Here's how the part is built. I have some questions about the finished solid (model axes, mm). A direction names the side the tool comes from. Round coordinates to 2 decimals unless told otherwise and drop trailing zeros. Write each loop counter-clockwise with the first axis right and the second up, starting at its lowest first coordinate (ties: lowest second). Pieces come first, ordered by that corner, then holes. Notation, with made-up numbers: (-27, 36.5) - (15, 36.5) arc R13 cw to (15, 49.5) - close; hole circle Ø3 at (1, 21.5). An arc over 180 degrees is marked (long way). One line per question, with ' | ' between items. Start each with the question number.
(1) Imagine slicing it at C-C (y = 147). Write out the boundary of the cut face in (x, z), plus the area to 3 significant figures.
(2) For faces 1 (the flat face through (30, 142, 24)), 2 (the flat face through (29, 149, 42)), 3 (the flat face through (32, -5, 45)), 4 (the flat face through (32, 147, 45)), which set-ups out of +Z, -Z, +X, -X, +Y, -Y let a thin tool reach every point of the face, with its end or its side?
(3) Imagine slicing it at D-D (z = 32). Write out the boundary of the cut face in (x, y), plus the area to 3 significant figures.
(4) Imagine slicing it at B-B (x = 29). Give the number of separate pieces and of enclosed holes in the cut face, plus the area to 3 significant figures.
(5) Will these pins go through, and if not, where does the flat tip stop? pin 1 (10 mm diameter, centred on x = 37.5, z = 42, fed in from +Y); pin 2 (3.5 mm diameter, centred on x = 29, y = 147, fed in from +Z); pin 3 (6 mm diameter, centred on x = 14, z = 15.5, fed in from -Y); pin 4 (1 mm diameter, centred on y = 89, z = 21, fed in from -X).
(6) Thinking about a two-plate mould opening in Y: for faces 5 (the flat face through (26, 147, 44)), 6 (the flat face through (30, -2, 23)), 7 (the flat face through (60, 72, 24)), which applies, pulls with the +Y half, pulls with the -Y half, needs draft (parallel to the pull), parting line crosses it, or undercut?
(7) If I drill on L1, parallel to Y at x = 29, z = 45.4; L2, parallel to Y at x = 21, z = 23; L3, parallel to X at y = 147, z = 43.6, over which ranges is the centre line in solid material (lowest first)?
(8) Imagine slicing it at A-A (z = 12). Write out the boundary of the cut face in (x, y).
Autodesk Inventor part; units mm, degrees
ref_plane "YZ Plane" through (0, 0, 0) normal (1, 0, 0) x (0, 1, 0)
ref_plane "XZ Plane" through (0, 0, 0) normal (0, 1, 0) x (-1, 0, 0)
ref_plane "XY Plane" through (0, 0, 0) normal (0, 0, 1) x (1, 0, 0)
sketch "Esboço1" plane through (0, 0, 0) normal (0, 0, 1) x (1, 0, 0)
  line L0 (0, 0) -> (60, 0)
  line L1 (60, 0) -> (60, 110)
  line L2 (60, 110) -> (0, 110)
  line L3 (0, 110) -> (0, 0)
  line L4 (62, 112) -> (62, -2)
  line L5 (62, -2) -> (-2, -2)
  line L6 (-2, -2) -> (-2, 112)
  line L7 (-2, 112) -> (62, 112)
  dimension "d0" = 60
  dimension "d1" = 110
  dimension "d2" = 2
extrude "Extrusão1" add sketch "Esboço1" along normal blind 2 contours L3 L2 L1 L0 | L4 L5 L6 L7
sketch "Esboço2" plane through (0, 0, 2) normal (0, 0, 1) x (1, 0, 0)
  line L0 (62, 112) -> (-2, 112)
  line L1 (-2, 112) -> (-2, -2)
  line L2 (62, -2) -> (62, 112)
  line L3 (-2, -2) -> (62, -2)
  line L4 (0, 0) -> (0, 110)
  line L5 (0, 110) -> (60, 110)
  line L6 (60, 110) -> (60, 0)
  line L7 (60, 0) -> (0, 0)
  point P0 (0, 0)
  dimension "d5" = 2
extrude "Extrusão2" add sketch "Esboço2" along normal blind 45
sketch "Esboço3" plane through (-2, -2, 0) normal (0, -1, 0) x (1, 0, 0)
  line L0 (45, 5) -> (57, 5)
  line L1 (57, 5) -> (57, 15)
  line L2 (57, 15) -> (45, 15)
  line L3 (45, 15) -> (45, 5)
  line L4 (0, 0) -> (64, 0)
  line L5 (64, 0) -> (64, 47)
  point P0 (2, 0)
  dimension "d8" = 10
  dimension "d9" = 12
  dimension "d10" = 5
  dimension "d11" = 7
extrude "Extrusão3" cut sketch "Esboço3" against normal blind 38
sketch "Esboço11" plane through (-2, 112, 0) normal (0, 1, 0) x (1, 0, 0)
  line L0 (64, 0) -> (64, -47)
  line L1 (0, 0) -> (64, 0)
  line L2 (64, 0) -> (64, -2)
  line L3 (64, -2) -> (0, -2)
  line L4 (0, -2) -> (0, 0)
  line L5 (64, 0) -> (0, 0)
  point P0 (2, 0)
  dimension "d45" = 2
  dimension "d46" = 0
  dimension "d47" = 64
extrude "Extrusão8" add sketch "Esboço11" along normal blind 32
sketch "Esboço18" plane through (-2, 112, 2) normal (0, 0, 1) x (1, 0, 0)
  line L0 (0, 0) -> (64, 0)
  line L1 (64, 32) -> (64, 0)
  line L2 (0, 32) -> (64, 32)
  line L3 (0, 0) -> (0, 32)
  line L4 (0, -114) -> (0, 0)
  line L5 (64, -114) -> (0, -114)
  line L6 (64, 0) -> (64, -114)
  line L7 (2, -112) -> (62, -112)
  line L8 (62, -112) -> (62, -2)
  line L9 (62, -2) -> (2, -2)
  line L10 (2, -2) -> (2, -112)
  line L11 (62, 0) -> (62, 30)
  line L12 (62, 30) -> (2, 30)
  line L13 (2, 30) -> (2, 0)
  dimension "d89" = 2
extrude "Extrusão15" add sketch "Esboço18" along normal blind 45 contours L3 L2 L1 L0 L11 L12 L13
sketch "Esboço20" plane through (-2, -2, 0) normal (-1, 0, 0) x (0, 0, 1)
  line L0 (25, 86) -> (15, 86)
  line L1 (15, 86) -> (15, 96)
  line L2 (15, 96) -> (25, 96)
  line L3 (25, 96) -> (25, 86)
  line L4 (0, 146) -> (47, 146)
  line L5 (0, 146) -> (0, 0)
  point P0 (0, 2)
  dimension "d101" = 10
  dimension "d102" = 10
  dimension "d103" = 50
  dimension "d104" = 15
extrude "Extrusão17" cut sketch "Esboço20" against normal blind 2
sketch "Esboço21" plane through (-2, -2, 0) normal (0, -1, 0) x (1, 0, 0)
  line L0 (62, 47) -> (2, 47)
  line L1 (28, 47) -> (34, 47)
  line L2 (34, 47) -> (34, 42)
  line L3 (34, 42) -> (28, 42)
  line L4 (28, 42) -> (28, 47)
  line L5 (64, 0) -> (64, 47)
  point P0 (2, 0)
  dimension "d108" = 6
  dimension "d109" = 5
  dimension "d110" = 30
extrude "Extrusão18" add sketch "Esboço21" along normal blind 6
sketch "Esboço22" plane through (0, 0, 47) normal (0, 0, 1) x (1, 0, 0)
  circle A0 centre (29, -5) radius 1.5
  line L0 (32, -2) -> (32, -8)
  line L1 (32, -8) -> (26, -8)
  point P0 (0, 0)
  dimension "d113" = 3
  dimension "d114" = 3
  dimension "d115" = 3
extrude "Extrusão19" cut sketch "Esboço22" against normal blind 6
sketch "Esboço23" plane through (-2, 144, 0) normal (0, 1, 0) x (1, 0, 0)
  line L0 (64, 0) -> (64, -47)
  line L1 (64, -47) -> (0, -47)
  line L2 (0, -47) -> (0, 0)
  line L3 (0, 0) -> (64, 0)
  line L4 (34, -42) -> (28, -42)
  line L5 (28, -42) -> (28, -47)
  line L6 (34, -47) -> (34, -42)
  point P0 (2, 0)
extrude "Extrusão20" add sketch "Esboço23" along normal blind 6 contours L1 L5 L4 L6
sketch "Esboço24" plane through (0, 0, 47) normal (0, 0, 1) x (1, 0, 0)
  circle A0 centre (29, 147) radius 1.5
  line L0 (26, 150) -> (32, 150)
  line L1 (32, 144) -> (32, 150)
  point P0 (0, 0)
  dimension "d120" = 3
  dimension "d121" = 3
  dimension "d122" = 3
extrude "Extrusão21" cut sketch "Esboço24" against normal blind 6
chamfer "Chanfro2" distance 1.5 angle 45 2 edges at (29, 144, 42) (29, -2, 42)
sketch "Esboço25" plane through (0, 0, 47) normal (0, 0, 1) x (1, 0, 0)
  line L0 (0, 0) -> (0, 110)
  line L1 (0, 110) -> (60, 110)
  line L2 (60, 110) -> (60, 112)
  line L3 (60, 112) -> (0, 112)
  line L4 (0, 112) -> (0, 110)
extrude "Extrusão22" cut sketch "Esboço25" against normal blind 45
sketch "Esboço26" plane through (-2, -2, 0) normal (0, -1, 0) x (1, 0, 0)
  line L0 (15, 3) -> (28, 3)
  line L1 (28, 3) -> (28, 15)
  line L2 (28, 15) -> (15, 15)
  line L3 (15, 15) -> (15, 3)
  line L4 (0, 0) -> (0, 47)
  line L5 (0, 0) -> (64, 0)
  point P0 (2, 0)
  dimension "d130" = 13
  dimension "d131" = 12
  dimension "d132" = 15
  dimension "d133" = 3
extrude "Extrusão23" cut sketch "Esboço26" against normal blind 10
properties part number "basecaixa"
Check sheet entries:
1) outline: (26, 42) - (27.5, 42) - (27.5, 47) - (26, 47) - close; (30.5, 42) - (32, 42) - (32, 47) - (30.5, 47) - close | area: 15.0 mm^2
2) face 1: +Z | face 2: -Z, +X, -X, +Y | face 3: +Z, -Z, +X, -Y | face 4: +Z, -Z, +X, +Y
3) outline: (-2, -2) - (62, -2) - (62, 144) - (-2, 144) - close; hole (0, 0) - (60, 0) - (60, 142) - (0, 142) - close | area: 824 mm^2
4) separate pieces: 3 | enclosed holes: 0 | area: 504 mm^2
5) pin 1: y = 144 | pin 2: z = 47 | pin 3: y = -2 | pin 4: x = 60
6) face 5: needs draft | face 6: pulls with the -Y half | face 7: undercut
7) L1: -8 to -6.5, -3.5 to 0, 142 to 145.5, 148.5 to 150 | L2: -2 to 0, 142 to 144 | L3: 26 to 27.5, 30.5 to 32
8) outline: (-2, -2) - (13, -2) - (13, 0) - (0, 0) - (0, 142) - (60, 142) - (60, 0) - (55, 0) - (55, -2) - (62, -2) - (62, 144) - (-2, 144) - close; (26, -2) - (43, -2) - (43, 0) - (26, 0) - close
